Drawing for the job (mm, zero at the part's lowest x, y, z). A direction names the side the tool comes from. Give positions to 0.01 mm unless a question says otherwise; leave off trailing zeros. Write each loop counter-clockwise with the first axis right and the second up, starting at its lowest first coordinate (ties: lowest second). Pieces come first, ordered by that corner, then holes. Notation, with made-up numbers: M 24,-0.75 L 62,-0.75 A13 cw 62,4.25 Z; hole C -34.5,35.5 d10. An arc over 180 degrees is marked long. Use CSV: the item, a comma, the result in double quotes. Start each with the question number.
1. Band-saw the part on A-A, the plane x = 21. List the corners of the cut face in (y, z).
2. Drop flat-ended pins along their axis: pin 1 Ø13 at (x, z) = (20.5, 17.5) entering from -Y; pin 2 Ø16 at (x, y) = (23, 39) entering from -Z. Give the stop position or say it passes through.
3. Mould opens along X. For the marked faces 1, 2 and 3 say: pulls with the +X half, pulls with the -X half, needs draft (parallel to the pull), parting line crosses it, or undercut.
4. Band-saw the part on B-B, the plane z = 16. List the corners of the cut face in (x, y).
5. Band-saw the part on C-C, the plane x = 6.5. List the corners of the cut face in (y, z).
6. Drill centre lines: line 1 along X through (y, z) = (61, 16); line 2 along Y through (x, z) = (15.5, 8.5); line 3 along Z through (x, y) = (29, 35.5). Where is each one in solid material? Low to high. Write a range as from..to.
7. 3-axis set-ups, long thin cutter, end or side, ignore diameter. For the marked faces 4, 5 and 6: which of +Z, -Z, +X, -X, +Y, -Y reach the whole face in a straight line?
8. Band-saw the part on D-D, the plane y = 39.5. List the corners of the cut face in (x, z).
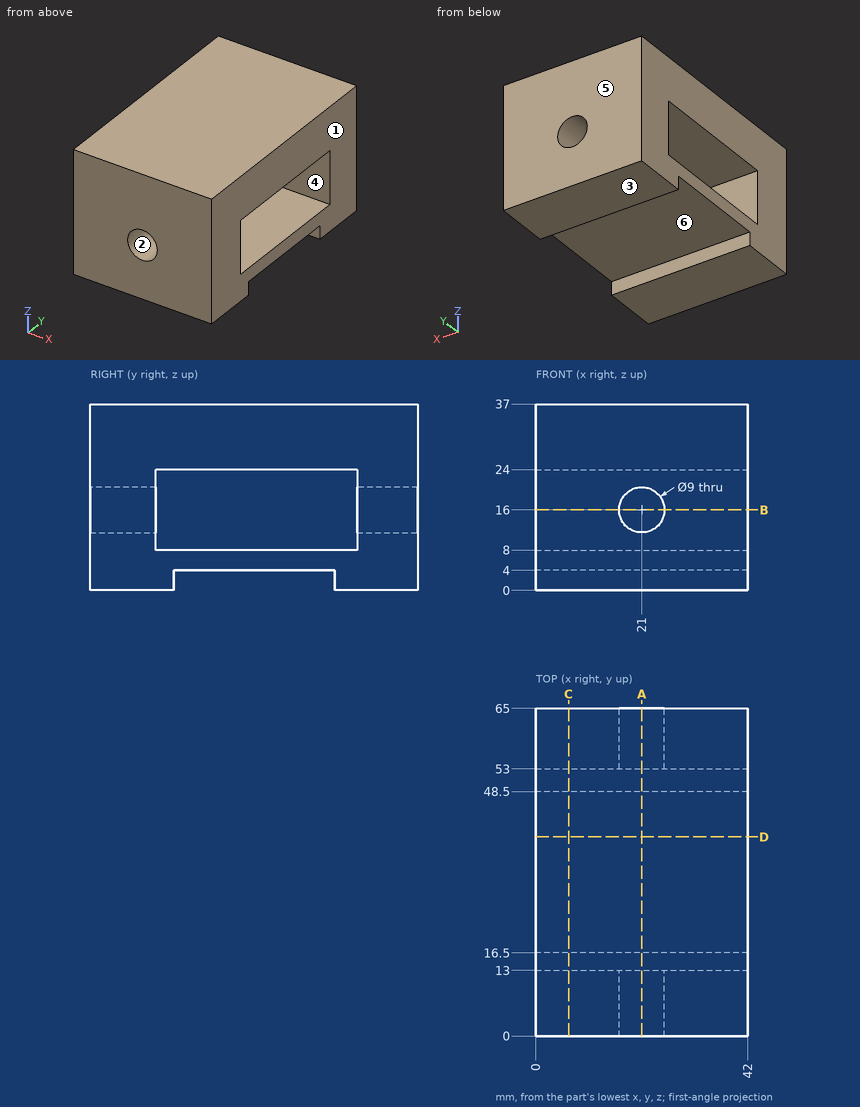
Output:
1,outline,"M 0,0 L 16.5,0 L 16.5,4 L 48.5,4 L 48.5,0 L 65,0 L 65,11.5 L 53,11.5 L 53,8 L 13,8 L 13,11.5 L 0,11.5 Z; M 0,20.5 L 13,20.5 L 13,24 L 53,24 L 53,20.5 L 65,20.5 L 65,37 L 0,37 Z"
2,pin 1,"stops at y = 0"
2,pin 2,"stops at z = 4"
3,face 1,"pulls with the +X half"
3,face 2,"undercut"
3,face 3,"needs draft"
4,outline,"M 0,0 L 16.5,0 L 16.5,13 L 0,13 Z; M 0,53 L 16.5,53 L 16.5,65 L 0,65 Z; M 25.5,0 L 42,0 L 42,13 L 25.5,13 Z; M 25.5,53 L 42,53 L 42,65 L 25.5,65 Z"
5,outline,"M 0,0 L 16.5,0 L 16.5,4 L 48.5,4 L 48.5,0 L 65,0 L 65,37 L 0,37 Z; hole M 13,8 L 53,8 L 53,24 L 13,24 Z"
6,line 1,"x = 0..16.5, 25.5..42"
6,line 2,"y = 0..13, 53..65"
6,line 3,"z = 4..8, 24..37"
7,face 4,"+X, -X"
7,face 5,"+Z, -Z, +X, -X, +Y"
7,face 6,"-Z, +X, -X"
8,outline,"M 0,4 L 42,4 L 42,8 L 0,8 Z; M 0,24 L 42,24 L 42,37 L 0,37 Z"
